Verification items for the finished model (mm, model axes). A direction names the side the tool comes from. Coordinates: 2 decimals unless noted, no trailing zeros. Order: outer loops, then holes, each group sorted by start corner. A loop starts at its lowest first (then second) coordinate and runs counter-clockwise, first axis right, second up. Notation, with made-up numbers: (-16.75, 11) -> (11.25, 11) arc R33 cw to (11.25, 41) -> close; hole circle Ø5 at (51, -13). An arc over 180 degrees is marked (long way). Write each question's results on one line, items separated by ' | '. Start each with the question number.
(1) Set-up check for faces 1 (the flat face through (74.5, 41.483, 15.1)), 2 (the flat face through (11, 14, 3)), 3 (the cylindrical face through (64.553, 7.813, 1.479)): record each of +Z, -Z, +X, -X, +Y, -Y from which the full face is reachable in a straight line by a thin tool's end or side.
(2) Cross-section at C-C on y = -2. Enter the section's corners in (x, z).
(3) Cross-section at A-A on x = -1. Enter the section's corners in (y, z), and give its area (3 significant figures).
(4) Go/stop test with flat-tipped pins: pin 1 (3.5 mm diameter, centred on x = -5, z = 2, fed in from +Y); pin 2 (8 mm diameter, centred on x = 59.5, z = 50.5, fed in from +Y); pin 3 (2 mm diameter, centred on x = 54, y = 30.5, fed in from -Z). Record where each tip stops, or that it passes through.
(5) Cross-section at D-D on y = 33.5. Enter the section's corners in (x, z), and give its area (3 significant figures).
(6) Draft check along Z on faces 4 (the flat face through (11, 9, 0)), 5 (the flat face through (11, 14, 147)), 6 (the flat face through (11, 9, 150)). Enter one of: +Z half, -Z half, draft (parallel to the pull), parting line (faces both ways), or undercut.
(7) Cross-section at B-B on z = 64. Enter the section's corners in (x, y), and give its area (3 significant figures).
(8) Thickness scan on probe 1 along X at (y, z) = (5, 18.5); probe 2 along Z at (x, y) = (15.5, -10); probe 3 along Y at (x, z) = (13.5, 8.5). Record the ranges inside material, lowest first. Write a range as [from, to].
```python
from build123d import *

# Parameters (mm, degrees)
ESBO_O1_W                = 130
ESBO_O1_H                = 65
RESSALTO_EXTRUS_O1_DEPTH = 150
ESBO_O2_W                = 70
ESBO_O2_H                = 10
CORTE_EXTRUS_O1_DEPTH    = 131
ESBO_O3_W                = 40
ESBO_O3_H                = 3
CORTE_EXTRUS_O2_DEPTH    = 131
ESBO_O4_W                = 40
ESBO_O4_H                = 3
CORTE_EXTRUS_O3_DEPTH    = 151
ESBO_O5_R                = 7.5
ESBO_O5_W                = 20
ESBO_O5_H                = 10
CORTE_EXTRUS_O4_DEPTH    = 141
ESBO_O6_W                = 124
ESBO_O6_H                = 144
CORTE_EXTRUS_O5_DEPTH    = 55
ESBO_O9_W                = 23
ESBO_O9_H                = 12
CORTE_EXTRUS_O6_DEPTH    = 3


with BuildPart() as part:
    # Esboço1 → Ressalto-extrusão1 (new body)
    with BuildSketch(Plane.XY):
        with Locations((12.060242954, 8.983357453)):
            Rectangle(ESBO_O1_W, ESBO_O1_H)
    extrude(amount=RESSALTO_EXTRUS_O1_DEPTH)

    # Esboço2 → Corte-extrusão1 (cut, through all)
    with BuildSketch(Plane.ZY.offset(52.939757046)):
        with Locations((85, -3.516642547)):
            Rectangle(ESBO_O2_W, ESBO_O2_H)
    extrude(amount=-CORTE_EXTRUS_O1_DEPTH, mode=Mode.SUBTRACT)

    # Esboço3 → Corte-extrusão2 (cut, through all)
    with BuildSketch(Plane.ZY.offset(52.939757046)):
        with Locations((75, 39.983357453)):
            Rectangle(ESBO_O3_W, ESBO_O3_H)
    extrude(amount=-CORTE_EXTRUS_O2_DEPTH, mode=Mode.SUBTRACT)

    # Esboço4 → Corte-extrusão3 (cut, through all)
    with BuildSketch(Plane(origin=(0, 0, 0), x_dir=(-1, 0, 0), z_dir=(0, 0, -1))):
        with Locations((-12.060242954, 39.983357453)):
            Rectangle(ESBO_O4_W, ESBO_O4_H)
    extrude(amount=-CORTE_EXTRUS_O3_DEPTH, mode=Mode.SUBTRACT)

    # Esboço5 → Corte-extrusão4 (cut)
    with BuildSketch(Plane(origin=(0, 0, 0), x_dir=(-1, 0, 0), z_dir=(0, 0, -1))):
        with Locations((-57.060242954, 7.483357453)):
            Circle(ESBO_O5_R)
        with Locations((7.939757046, 12.483357453)):
            Rectangle(ESBO_O5_W, ESBO_O5_H)
    extrude(amount=-CORTE_EXTRUS_O4_DEPTH, mode=Mode.SUBTRACT)

    # Esboço6 → Corte-extrusão5 (cut)
    with BuildSketch(Plane(origin=(0, 41.483357453, 0), x_dir=(1, 0, 0), z_dir=(0, 1, 0))):
        with Locations((12.060242954, -75)):
            Rectangle(ESBO_O6_W, ESBO_O6_H)
    extrude(amount=-CORTE_EXTRUS_O5_DEPTH, mode=Mode.SUBTRACT)

    # Esboço9 → Corte-extrusão6 (cut)
    with BuildSketch(Plane(origin=(0, 0, 0), x_dir=(-1, 0, 0), z_dir=(0, 0, -1))):
        with Locations((-34.560242954, 13.483357453)):
            Rectangle(ESBO_O9_W, ESBO_O9_H)
    extrude(amount=-CORTE_EXTRUS_O6_DEPTH, mode=Mode.SUBTRACT)


solid = part.part
```
Results are:
1) face 1: +Z, -Z, +X, -X, +Y | face 2: +Y | face 3: -Z
2) outline: (-52.94, 0) -> (77.06, 0) -> (77.06, 50) -> (74.06, 50) -> (74.06, 3) -> (-49.94, 3) -> (-49.94, 50) -> (-52.94, 50) -> close; (-52.94, 120) -> (-49.94, 120) -> (-49.94, 147) -> (74.06, 147) -> (74.06, 120) -> (77.06, 120) -> (77.06, 150) -> (-52.94, 150) -> close
3) outline: (-23.52, 0) -> (7.48, 0) -> (7.48, 3) -> (-13.52, 3) -> (-13.52, 147) -> (38.48, 147) -> (38.48, 150) -> (-23.52, 150) -> close; (17.48, 0) -> (38.48, 0) -> (38.48, 3) -> (17.48, 3) -> close | area: 1,780 mm2
4) pin 1: stops at y = 38.48 | pin 2: stops at y = -13.52 | pin 3: stops at z = 0
5) outline: (-52.94, 0) -> (77.06, 0) -> (77.06, 150) -> (-52.94, 150) -> close; hole (-49.94, 3) -> (74.06, 3) -> (74.06, 147) -> (-49.94, 147) -> close | area: 1,640 mm2
6) face 4: -Z half | face 5: undercut | face 6: +Z half
7) outline: (-52.94, -23.52) -> (77.06, -23.52) -> (77.06, -8.52) -> (74.06, -8.52) -> (74.06, -13.52) -> (-49.94, -13.52) -> (-49.94, -8.52) -> (-52.94, -8.52) -> close; (-52.94, 1.48) -> (-49.94, 1.48) -> (-49.94, 38.48) -> (-52.94, 38.48) -> close; (74.06, 1.48) -> (77.06, 1.48) -> (77.06, 38.48) -> (74.06, 38.48) -> close | area: 1,550 mm2
8) probe 1: x = [-52.94, -49.94], [74.06, 77.06] | probe 2: z = [0, 3], [147, 150] | probe 3: y = [-23.52, -13.52]
